For this review, take the finished solid that the model builds, in its own axes (mm). A direction names the side the tool comes from. Give positions to 0.01 mm unless a question says otherwise; leave off trailing zeros. Loops run counter-clockwise (first coordinate to the right, second up) from the corner with the lowest first, then second, coordinate; pieces in that order, holes last. Notation, with made-up numbers: (30, -34.5) - (68, -34.5) arc R12 cw to (68, -23.5) - close; hole circle Ø11 at (-22.5, 54.5). An arc over 180 degrees is marked (long way). Answer in a Markdown table with one row per item.
```python
from build123d import *

# Parameters (mm, degrees)
SKETCH1_R                = 11.1
BOSS_EXTRUDE1_DEPTH      = 3.6
BOSS_EXTRUDE2_DEPTH      = 1.7
BOSS_EXTRUDE2_DEPTH_BACK = 13.3
SKETCH2_R                = 5.15
SKETCH3_R                = 4
SKETCH3_R_2              = 2
CUT_EXTRUDE1_DEPTH       = 22.712208547


with BuildPart() as part:
    # Sketch1 → Boss-Extrude1 (new body)
    with BuildSketch(Plane(origin=(0, 0, 0), x_dir=(1, 0, 0), z_dir=(0, 1, 0))):
        with Locations(Location((0, 0, 0), (0, 0, 270))):
            Circle(SKETCH1_R)
    extrude(amount=BOSS_EXTRUDE1_DEPTH)

    # Sketch2 → Boss-Extrude2 (add, two sides: drawn at the far end of the back side and taken through both)
    with BuildSketch(Plane(origin=(0, 3.6, 0), x_dir=(1, 0, 0), z_dir=(0, 1, 0)).offset(-BOSS_EXTRUDE2_DEPTH_BACK)):
        with Locations(Location((0, 0, 0), (0, 0, 270))):
            Circle(SKETCH2_R)
    extrude(amount=BOSS_EXTRUDE2_DEPTH + BOSS_EXTRUDE2_DEPTH_BACK)

    # Sketch3 → Cut-Extrude1 (cut, through all)
    with BuildSketch(Plane(origin=(0, 5.3, 0), x_dir=(1, 0, 0), z_dir=(0, 1, 0))):
        with Locations(Location((0, 0, 0), (0, 0, 270))):
            Circle(SKETCH3_R)
        with Locations(Location((-8.1, 0, 0), (0, 0, 270))):
            Circle(SKETCH3_R_2)
        with Locations(Location((8.1, 0, 0), (0, 0, 270))):
            Circle(SKETCH3_R_2)
        with Locations(Location((0, 8.1, 0), (0, 0, 270))):
            Circle(SKETCH3_R_2)
        with Locations(Location((0, -8.1, 0), (0, 0, 270))):
            Circle(SKETCH3_R_2)
    extrude(amount=-CUT_EXTRUDE1_DEPTH, mode=Mode.SUBTRACT)


solid = part.part
```
1. We need section B-B, the plane z = 8.1. Give the boundary of the cut face in (x, y), and give its area (3 significant figures).
Values:
| item | result |
|---|---|
| outline | (-7.59, 0) - (-2, 0) - (-2, 3.6) - (-7.59, 3.6) - close; (2, 0) - (7.59, 0) - (7.59, 3.6) - (2, 3.6) - close |
| area | 40.2 mm^2 |
2. We need section A-A, the plane x = -3. Give the boundary of the cut face in (y, z).
Values:
| item | result |
|---|---|
| outline | (-9.7, -4.19) - (0, -4.19) - (0, -10.69) - (3.6, -10.69) - (3.6, -4.19) - (5.3, -4.19) - (5.3, -2.65) - (-9.7, -2.65) - close; (-9.7, 2.65) - (5.3, 2.65) - (5.3, 4.19) - (3.6, 4.19) - (3.6, 10.69) - (0, 10.69) - (0, 4.19) - (-9.7, 4.19) - close |
3. We need section C-C, the plane x = 0.75. Give the boundary of the cut face in (y, z).
Values:
| item | result |
|---|---|
| outline | (-9.7, -5.1) - (0, -5.1) - (0, -6.25) - (3.6, -6.25) - (3.6, -5.1) - (5.3, -5.1) - (5.3, -3.93) - (-9.7, -3.93) - close; (-9.7, 3.93) - (5.3, 3.93) - (5.3, 5.1) - (3.6, 5.1) - (3.6, 6.25) - (0, 6.25) - (0, 5.1) - (-9.7, 5.1) - close; (0, -11.07) - (3.6, -11.07) - (3.6, -9.95) - (0, -9.95) - close; (0, 9.95) - (3.6, 9.95) - (3.6, 11.07) - (0, 11.07) - close |
4. Clearance check with flat-ended pins moving along their axes: pin 1 (4.5 mm diameter, centred on x = 0, z = 8.1, fed in from +Y); pin 2 (1 mm diameter, centred on x = 6.5, y = 1, fed in from +Z); pin 3 (2 mm diameter, centred on x = -5.5, y = -2.5, fed in from +Z). State where each tip first meets the part, or that it passes through.
Values:
| item | result |
|---|---|
| pin 1 | stops at y = 3.6 |
| pin 2 | stops at z = 9.34 |
| pin 3 | stops at z = 2.5 |
5. We need section D-D, the plane y = 1.5. Give the boundary of the cut face in (x, z), and give its area (3 significant figures).
Values:
| item | result |
|---|---|
| outline | circle Ø22.2 at (0, 0); hole circle Ø4 at (-8.1, 0); hole circle Ø8 at (0, 0); hole circle Ø4 at (0, -8.1); hole circle Ø4 at (0, 8.1); hole circle Ø4 at (8.1, 0) |
| area | 287 mm^2 |
6. Wall thickness on line 1 (X direction, y = 1.6, z = 0); line 2 (X direction, y = 2, z = -1.75); line 3 (Y direction, x = 5.75, z = -7.5): over which ranges is each line inside the solid? List them lowest first. Write a range as [from, to].
Values:
| item | result |
|---|---|
| line 1 | x = [-11.1, -10.1], [-6.1, -4], [4, 6.1], [10.1, 11.1] |
| line 2 | x = [-10.96, -9.07], [-7.13, -3.6], [3.6, 7.13], [9.07, 10.96] |
| line 3 | y = [0, 3.6] |
7. For faces 1 (the face through (-2, 3.6, 5)), 2 (the face through (-3.905, -2.095, -0.867)), 3 (the face through (-2, 0, 5)), list the 3-axis set-ups (+Z, -Z, +X, -X, +Y, -Y) from which the entire face can be reached by the end or side of a thin tool; tool diameter is ignored.
Values:
| item | result |
|---|---|
| face 1 | +Y |
| face 2 | +Y, -Y |
| face 3 | -Y |
